Input: part model. Units: mm. Frame: model coordinates. Give positions to 0.01 mm unless a question says otherwise; leave off trailing zeros. Loops run counter-clockwise (first coordinate to the right, second up) from the corner with the lowest first, then second, coordinate; pieces in that order, holes last. Notation, with made-up numbers: M 40.5,-5 L 68.5,-5 A21 ccw 68.5,13 Z; hole C -22,14 d3. An arc over 180 degrees is marked long. Return JSON: item names as keys, results as strings. Group by question number.
```python
from build123d import *

# Parameters (mm, degrees)
SKETCH1_W           = 209.55
SKETCH1_H           = 139.7
SKETCH1_W_2         = 203.2
SKETCH1_H_2         = 133.35
BOSS_EXTRUDE1_DEPTH = 101.6
SKETCH2_W           = 209.55
SKETCH2_H           = 139.7
BOSS_EXTRUDE2_DEPTH = 3.175
SKETCH3_R           = 2.54
CUT_EXTRUDE1_DEPTH  = 162.800442289
SKETCH4_W           = 209.55
SKETCH4_H           = 139.7
BOSS_EXTRUDE3_DEPTH = 3.175


with BuildPart() as part:
    # Sketch1 → Boss-Extrude1 (new body)
    with BuildSketch(Plane(origin=(0, 0, 0), x_dir=(1, 0, 0), z_dir=(0, 1, 0))):
        Rectangle(SKETCH1_W, SKETCH1_H)
        Rectangle(SKETCH1_W_2, SKETCH1_H_2, mode=Mode.SUBTRACT)
    extrude(amount=BOSS_EXTRUDE1_DEPTH)

    # Sketch2 → Boss-Extrude2 (add)
    with BuildSketch(Plane(origin=(0, 0, 0), x_dir=(1, 0, 0), z_dir=(0, 1, 0))):
        Rectangle(SKETCH2_W, SKETCH2_H)
    extrude(amount=-BOSS_EXTRUDE2_DEPTH)

    # Sketch3 → Cut-Extrude1 (cut, through all)
    with BuildSketch(Plane(origin=(0, 0, 0), x_dir=(1, 0, 0), z_dir=(0, 1, 0))):
        with Locations(Location((-76.2, 50.8, 0), (0, 0, 270))):
            Circle(SKETCH3_R)
        with Locations(Location((-63.5, 50.8, 0), (0, 0, 270))):
            Circle(SKETCH3_R)
        with Locations(Location((-50.8, 50.8, 0), (0, 0, 270))):
            Circle(SKETCH3_R)
        with Locations(Location((-38.1, 50.8, 0), (0, 0, 270))):
            Circle(SKETCH3_R)
        with Locations(Location((-63.5, 38.1, 0), (0, 0, 270))):
            Circle(SKETCH3_R)
        with Locations(Location((-50.8, 38.1, 0), (0, 0, 270))):
            Circle(SKETCH3_R)
        with Locations(Location((-38.1, 38.1, 0), (0, 0, 270))):
            Circle(SKETCH3_R)
        with Locations(Location((-63.5, 25.4, 0), (0, 0, 270))):
            Circle(SKETCH3_R)
        with Locations(Location((-50.8, 25.4, 0), (0, 0, 270))):
            Circle(SKETCH3_R)
        with Locations(Location((-38.1, 25.4, 0), (0, 0, 270))):
            Circle(SKETCH3_R)
        with Locations(Location((-63.5, 12.7, 0), (0, 0, 270))):
            Circle(SKETCH3_R)
        with Locations(Location((-50.8, 12.7, 0), (0, 0, 270))):
            Circle(SKETCH3_R)
        with Locations(Location((-38.1, 12.7, 0), (0, 0, 270))):
            Circle(SKETCH3_R)
        with Locations(Location((-63.5, 0, 0), (0, 0, 270))):
            Circle(SKETCH3_R)
        with Locations(Location((-50.8, 0, 0), (0, 0, 270))):
            Circle(SKETCH3_R)
        with Locations(Location((-38.1, 0, 0), (0, 0, 270))):
            Circle(SKETCH3_R)
        with Locations(Location((-63.5, -12.7, 0), (0, 0, 270))):
            Circle(SKETCH3_R)
        with Locations(Location((-50.8, -12.7, 0), (0, 0, 270))):
            Circle(SKETCH3_R)
        with Locations(Location((-38.1, -12.7, 0), (0, 0, 270))):
            Circle(SKETCH3_R)
        with Locations(Location((-63.5, -25.4, 0), (0, 0, 270))):
            Circle(SKETCH3_R)
        with Locations(Location((-50.8, -25.4, 0), (0, 0, 270))):
            Circle(SKETCH3_R)
        with Locations(Location((-38.1, -25.4, 0), (0, 0, 270))):
            Circle(SKETCH3_R)
        with Locations(Location((-63.5, -38.1, 0), (0, 0, 270))):
            Circle(SKETCH3_R)
        with Locations(Location((-50.8, -38.1, 0), (0, 0, 270))):
            Circle(SKETCH3_R)
        with Locations(Location((-38.1, -38.1, 0), (0, 0, 270))):
            Circle(SKETCH3_R)
        with Locations(Location((-63.5, -50.8, 0), (0, 0, 270))):
            Circle(SKETCH3_R)
        with Locations(Location((-50.8, -50.8, 0), (0, 0, 270))):
            Circle(SKETCH3_R)
        with Locations(Location((-38.1, -50.8, 0), (0, 0, 270))):
            Circle(SKETCH3_R)
        with Locations(Location((-76.2, 38.1, 0), (0, 0, 270))):
            Circle(SKETCH3_R)
        with Locations(Location((-76.2, 25.4, 0), (0, 0, 270))):
            Circle(SKETCH3_R)
        with Locations(Location((-76.2, 12.7, 0), (0, 0, 270))):
            Circle(SKETCH3_R)
        with Locations(Location((-76.2, 0, 0), (0, 0, 270))):
            Circle(SKETCH3_R)
        with Locations(Location((-76.2, -12.7, 0), (0, 0, 270))):
            Circle(SKETCH3_R)
        with Locations(Location((-76.2, -25.4, 0), (0, 0, 270))):
            Circle(SKETCH3_R)
        with Locations(Location((-76.2, -38.1, 0), (0, 0, 270))):
            Circle(SKETCH3_R)
        with Locations(Location((-76.2, -50.8, 0), (0, 0, 270))):
            Circle(SKETCH3_R)
    extrude(amount=-CUT_EXTRUDE1_DEPTH, mode=Mode.SUBTRACT)

    # Sketch4 → Boss-Extrude3 (add)
    with BuildSketch(Plane.XZ.offset(3.175)):
        Rectangle(SKETCH4_W, SKETCH4_H)
    extrude(amount=BOSS_EXTRUDE3_DEPTH)


solid = part.part
```
Item 1: First-contact query: pin 1 Ø1 at (x, z) = (60, 38) entering from +Y; pin 2 Ø3 at (x, z) = (-76.2, 12.7) entering from +Y (3 decimals). Flat tips, straight axial feed; report the tip coordinate or a pass-through.
Item 2: Material intervals for line 1 (X direction, y = -2, z = -25.4) (3 decimals); line 2 (Z direction, x = 89, y = 39.5) (3 decimals); line 3 (X direction, y = 70, z = 19) (3 decimals), sorted ascending. Write a range as from..to.
Item 3: Section B-B, the plane y = 72. Return loops of the section in (x, z) (3 decimals), then the cut area to 3 significant figures.
Item 4: Section A-A, the plane z = 0. Return loops of the section in (x, y) (3 decimals), then the cut area to 3 significant figures.
Item 5: Section C-C, the plane x = -29. Return loops of the section in (y, z) (3 decimals).
Item 6: Section D-D, the plane z = 46. Return loops of the section in (x, y) (3 decimals).
Answer below:
{
 "1": {"pin 1": "y = 0", "pin 2": "y = -3.175"},
 "2": {"line 1": "-104.775..-78.74, -73.66..-66.04, -60.96..-53.34, -48.26..-40.64, -35.56..104.775", "line 2": "-69.85..-66.675, 66.675..69.85", "line 3": "-104.775..-101.6, 101.6..104.775"},
 "3": {"outline": "M -104.775,-69.85 L 104.775,-69.85 L 104.775,69.85 L -104.775,69.85 Z; hole M -101.6,-66.675 L 101.6,-66.675 L 101.6,66.675 L -101.6,66.675 Z", "area": "2,180 mm^2"},
 "4": {"outline": "M -104.775,-6.35 L 104.775,-6.35 L 104.775,101.6 L 101.6,101.6 L 101.6,0 L -35.56,0 L -35.56,-3.175 L -40.64,-3.175 L -40.64,0 L -48.26,0 L -48.26,-3.175 L -53.34,-3.175 L -53.34,0 L -60.96,0 L -60.96,-3.175 L -66.04,-3.175 L -66.04,0 L -73.66,0 L -73.66,-3.175 L -78.74,-3.175 L -78.74,0 L -101.6,0 L -101.6,101.6 L -104.775,101.6 Z", "area": "1,910 mm^2"},
 "5": {"outline": "M -6.35,-69.85 L 101.6,-69.85 L 101.6,-66.675 L 0,-66.675 L 0,66.675 L 101.6,66.675 L 101.6,69.85 L -6.35,69.85 Z"},
 "6": {"outline": "M -104.775,-6.35 L 104.775,-6.35 L 104.775,101.6 L 101.6,101.6 L 101.6,0 L -101.6,0 L -101.6,101.6 L -104.775,101.6 Z"}
}
